Here's the drawing with two shaded views (mm, measured from the low corner). I have some questions. A direction names the side the tool comes from. Give positions to 0.01 mm unless a question says otherwise; leave off trailing zeros. Loops run counter-clockwise (first coordinate to the right, second up) from the corner with the lowest first, then second, coordinate; pieces in that order, holes last. Notation, with made-up numbers: M 80.25,11.5 L 138.25,11.5 A15 cw 138.25,17.5 Z; hole C -19.75,53.5 d2. An arc over 180 degrees is marked long. Answer in a Markdown table with one row per item. Add a question column.
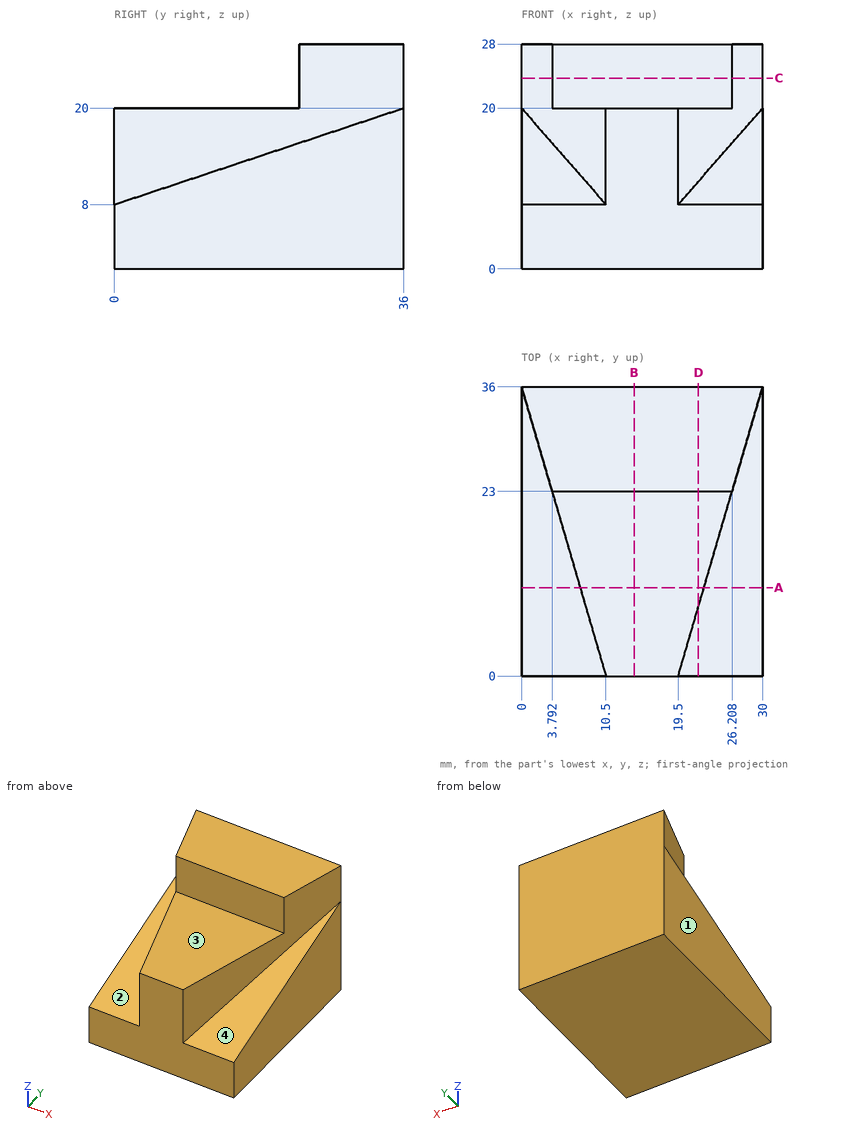
Item 1: Suppose I cut it at B-B (x = 14). List the corners of the cut face in (y, z) for me, then the cut area to 3 significant figures.
Item 2: Suppose I cut it at C-C (z = 23.75). List the corners of the cut face in (x, y) for me.
Item 3: Suppose I cut it at D-D (x = 22). List the corners of the cut face in (y, z) for me, then the cut area to 3 significant figures.
Item 4: I need wall thicknesses on L1, parallel to Z at x = 12, y = 12; L2, parallel to Y at x = 25, z = 25.75; L3, parallel to Z at x = 21, y = 3. Which ranges of each line are inside material? Lowest first, please.
Item 5: For the marked faces 1, 2, 3 and 4, which set-ups out of +Z, -Z, +X, -X, +Y, -Y let a thin tool reach every point of the face, with its end or its side?
Item 6: For P1, Ø10, axis at y = 16.5, z = 20.5, coming from the +X side; P2, Ø2.5, axis at x = 19.5, z = 25, coming from the -Y side; P3, Ø12, axis at x = 17, y = 7.5, coming from the +Z side, each with a flat end and sliding along its axis, tell me the tip position at first contact or that it passes through.
Item 7: Suppose I cut it at A-A (y = 11). List the corners of the cut face in (x, z) for me.
Values found:
| question | item | result |
|---|---|---|
| 1 | outline | M 0,0 L 36,0 L 36,28 L 23,28 L 23,20 L 0,20 Z |
| 1 | area | 824 mm² |
| 2 | outline | M 0,36 L 3.79,23 L 26.21,23 L 30,36 Z |
| 3 | outline | M 0,0 L 36,0 L 36,28 L 23,28 L 23,20 L 8.57,20 L 8.57,10.86 L 0,8 Z |
| 3 | area | 733 mm² |
| 4 | L1 | 0 to 20 |
| 4 | L2 | 23 to 36 |
| 4 | L3 | 0 to 9 |
| 5 | face 1 | +Z, -Z, -X, +Y, -Y |
| 5 | face 2 | +Z, -X, -Y |
| 5 | face 3 | +Z, +X, -X, -Y |
| 5 | face 4 | +Z, +X, -Y |
| 6 | P1 | x = 25.76 |
| 6 | P2 | y = 23 |
| 6 | P3 | z = 20 |
| 7 | outline | M 0,0 L 30,0 L 30,11.67 L 22.71,11.67 L 22.71,20 L 7.29,20 L 7.29,11.67 L 0,11.67 Z |
